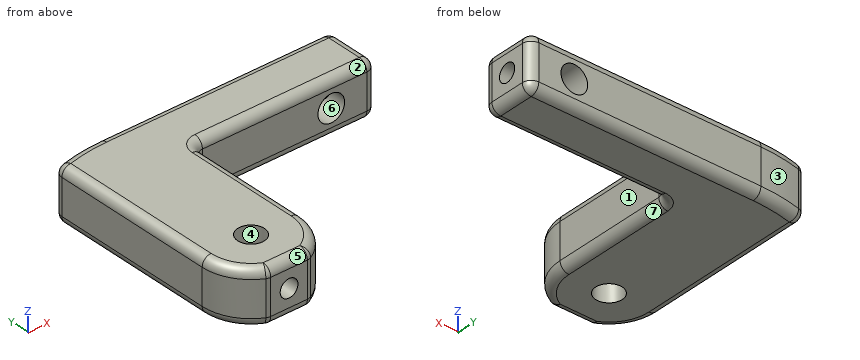
```python
from build123d import *

# Parameters (mm, degrees)
SKETCH_1_W          = 11
SKETCH_1_H          = 20
EXTRUDE_1_DEPTH     = 6
CUT_EXTRUDE_1_DEPTH = 6
SKETCH_3_R          = 5.5
EXTRUDE_2_DEPTH     = 6
SKETCH_4_W          = 24
SKETCH_4_H          = 6
EXTRUDE_3_DEPTH     = 6
SKETCH_6_R          = 1.5
CUT_EXTRUDE_3_DEPTH = 6
SKETCH_7_R          = 1.5
CUT_EXTRUDE_4_DEPTH = 6
SKETCH_5_W          = 6
SKETCH_5_H          = 0.5
CUT_EXTRUDE_5_DEPTH = 10
SKETCH_14_R         = 1
CUT_EXTRUDE_6_DEPTH = 4
SKETCH_15_W         = 6
SKETCH_15_H         = 6
EXTRUDE_4_DEPTH     = 2
SKETCH_16_R         = 1
CUT_EXTRUDE_7_DEPTH = 4
FILLET_2_R          = 1


# Read off the part's stored shape, not the designer's step: 切除-拉伸1
with BuildPart() as part:
    # 草图1 → 凸台-拉伸1 (new body)
    with BuildSketch(Plane.XY):
        with Locations((5.5, 10)):
            Rectangle(SKETCH_1_W, SKETCH_1_H)
    extrude(amount=EXTRUDE_1_DEPTH)

    # 切除-拉伸1 outline → 切除-拉伸1 (cut)
    with BuildSketch(Plane.XY):
        with BuildLine():
            Line((0, 20), (0, 19.228884523))
            ThreePointArc((0, 19.228884523), (2.723103392, 19.806282974), (5.5, 20))
            Line((5.5, 20), (0, 20))
        make_face()
        with BuildLine():
            Line((11, 20), (5.5, 20))
            ThreePointArc((5.5, 20), (8.276896608, 19.806282974), (11, 19.228884523))
            Line((11, 19.228884523), (11, 20))
        make_face()
    extrude(amount=CUT_EXTRUDE_1_DEPTH, mode=Mode.SUBTRACT)

    # 草图3 → 凸台-拉伸2 (add)
    with BuildSketch(Plane.XY):
        with Locations((5.5, 0)):
            Circle(SKETCH_3_R)
    extrude(amount=EXTRUDE_2_DEPTH)

    # 草图4 → 凸台-拉伸3 (add)
    with BuildSketch(Plane.XY):
        with Locations((17.5, 17)):
            Rectangle(SKETCH_4_W, SKETCH_4_H)
    extrude(amount=EXTRUDE_3_DEPTH)

    # 草图6 → 切除-拉伸3 (cut)
    with BuildSketch(Plane.XY):
        with Locations((5.5, 0)):
            Circle(SKETCH_6_R)
    extrude(amount=CUT_EXTRUDE_3_DEPTH, mode=Mode.SUBTRACT)

    # 草图7 → 切除-拉伸4 (cut)
    with BuildSketch(Plane.XZ.offset(-14)):
        with Locations((26.5, 3)):
            Circle(SKETCH_7_R)
    extrude(amount=-CUT_EXTRUDE_4_DEPTH, mode=Mode.SUBTRACT)

    # 草图5 → 切除-拉伸5 (cut)
    with BuildSketch(Plane.XY):
        with Locations((5.5, -5.25)):
            Rectangle(SKETCH_5_W, SKETCH_5_H)
    extrude(amount=CUT_EXTRUDE_5_DEPTH, mode=Mode.SUBTRACT)

    # 草图14 → 切除-拉伸6 (cut)
    with BuildSketch(Plane(origin=(0, -5, 0), x_dir=(-1, 0, 0), z_dir=(0, -1, 0))):
        with Locations(Location((-5.5, -3, 0), (0, 0, 90))):
            Circle(SKETCH_14_R)
    extrude(amount=-CUT_EXTRUDE_6_DEPTH, mode=Mode.SUBTRACT)

    # 草图15 → 凸台-拉伸4 (add)
    with BuildSketch(Plane(origin=(29.5, 0, 0), x_dir=(0, 0, -1), z_dir=(1, 0, 0))):
        with Locations((-3, 17)):
            Rectangle(SKETCH_15_W, SKETCH_15_H)
    extrude(amount=EXTRUDE_4_DEPTH)

    # 草图16 → 切除-拉伸7 (cut)
    with BuildSketch(Plane(origin=(31.5, 0, 0), x_dir=(0, 0, -1), z_dir=(1, 0, 0))):
        with Locations((-3, 17)):
            Circle(SKETCH_16_R)
    extrude(amount=-CUT_EXTRUDE_7_DEPTH, mode=Mode.SUBTRACT)

    # 圆角2
    fillet_2_edges = [part.edges().sort_by_distance(p)[0] for p in [
        (31.5, 17, 0),
        (31.5, 20, 3),
        (31.5, 17, 6),
        (31.5, 14, 3),
        (11, 7, 6),
        (0, 9.614442262, 0),
        (0, 9.614442262, 6),
        (0, 19.228884523, 3),
        (0.871172764, -2.970514841, 0),
        (0.871172764, -2.970514841, 6),
        (2.723103392, 19.806282974, 6),
        (2.723103392, 19.806282974, 0),
        (11, 14, 3),
        (11, 7, 0),
        (21.25, 14, 0),
        (21.25, 14, 6),
        (18.5, 20, 6),
        (18.5, 20, 0),
        (10.128827236, -2.970514841, 6),
        (10.128827236, -2.970514841, 0),
        (7.791287847, -5, 3),
        (3.208712153, -5, 3),
        (5.5, -5, 0),
        (5.5, -5, 6),
    ]]
    fillet(fillet_2_edges, radius=FILLET_2_R)


solid = part.part
```
Source: CAD feature listing. Evaluate the final solid. Frame: model axes, mm. Face numbers are marked on the shaded views. A direction names the side the tool comes from. Give positions to 0.01 mm unless a question says otherwise; leave off trailing zeros. Order: outer loops, then holes, each group sorted by start corner. A loop starts at its lowest first (then second) coordinate and runs counter-clockwise, first axis right, second up.
(1) Section query D-D (x = 12.5). Return the cut outline in (y, z), plus the area to 3 significant figures.
(2) Material intervals for line 1 along Y through (x, z) = (5.5, 1.75); line 2 along Z through (x, y) = (26.5, 16.25); line 3 along Z through (x, y) = (5.5, -2.5), sorted ascending.
(3) Section query C-C (y = 17). Return the cut outline in (x, z), plus the area to 3 significant figures.
(4) Section query A-A (x = 26.5). Return the cut outline in (y, z).
(5) Section query B-B (z = 3). Return the cut outline in (x, y), plus the area to 3 significant figures.
(6) Pull-direction query (X, two-part tool) for the marked faces 4, 5, 6 and 7; classes: +X half, -X half, draft (parallel to the pull), parting line (faces both ways), or undercut.
(7) Access query for the marked faces 1, 2 and 3. Directions: +Z, -Z, +X, -X, +Y, -Y. A direction counts if a zero-diameter tool reaches every point of the face in a straight line with its end or side. Return the directions, or none.
(8) Contact query for flat-ended pins moving along their axis: P1, Ø2, axis at y = 6.5, z = 3.5, coming from the +X side; P2, Ø1.2, axis at x = 17.5, z = 3.5, coming from the -Y side. Output: stop coordinate, or through.
Outcome:
1. outline: (14, 1) arc R1 ccw to (15, 0) - (19, 0) arc R1 ccw to (20, 1) - (20, 5) arc R1 ccw to (19, 6) - (15, 6) arc R1 ccw to (14, 5) - close
1. area: 35.1 mm2
2. line 1: y = -5 to -1.5, 1.5 to 20
2. line 2: z = 0 to 1.5, 4.5 to 6
2. line 3: z = 0 to 2, 4 to 6
3. outline: (0, 1) arc R1 ccw to (1, 0) - (30.5, 0) arc R1 ccw to (31.5, 1) - (31.5, 2) - (27.62, 2) arc R1.5 cw (long way) to (27.62, 4) - (31.5, 4) - (31.5, 5) arc R1 ccw to (30.5, 6) - (1, 6) arc R1 ccw to (0, 5) - close
3. area: 174 mm2
4. outline: (14, 1) arc R1 ccw to (15, 0) - (19, 0) arc R1 ccw to (20, 1) - (20, 1.5) - (14, 1.5) - close; (14, 4.5) - (20, 4.5) - (20, 5) arc R1 ccw to (19, 6) - (15, 6) arc R1 ccw to (14, 5) - close
5. outline: (0, 0) arc R5.5 ccw to (2.98, -4.89) arc R1 ccw to (3.44, -5) - (4.5, -5) - (4.5, -1.12) arc R1.5 cw (long way) to (6.5, -1.12) - (6.5, -5) - (7.56, -5) arc R1 ccw to (8.02, -4.89) arc R5.5 ccw to (11, 0) - (11, 13) arc R1 cw to (12, 14) - (25, 14) - (25, 20) - (5.5, 20) arc R20 ccw to (0.76, 19.43) arc R1 ccw to (0, 18.46) - close; (28, 14) - (30.5, 14) arc R1 ccw to (31.5, 15) - (31.5, 16) - (28, 16) - close; (28, 18) - (31.5, 18) - (31.5, 19) arc R1 ccw to (30.5, 20) - (28, 20) - close
5. area: 348 mm2
6. face 4: undercut
6. face 5: draft
6. face 6: undercut
6. face 7: +X half
7. face 1: +Z, -Z, +X, -Y
7. face 2: +Z, +X, -Y
7. face 3: +Z, -Z, -X, +Y
8. P1: stops at x = 11
8. P2: stops at y = 14
